from build123d import *

# Parameters (mm, degrees)
SKETCH1_R           = 4
BOSS_EXTRUDE1_DEPTH = 6
BOSS_EXTRUDE2_DEPTH = 6
CIRPATTERN1_COUNT   = 17
SKETCH5_R           = 3
CUT_EXTRUDE1_DEPTH  = 6


with BuildPart() as part:
    # Sketch1 → Boss-Extrude1 (new body)
    with BuildSketch(Plane.XY):
        Circle(SKETCH1_R)
    extrude(amount=BOSS_EXTRUDE1_DEPTH)

    # Sketch3 → Boss-Extrude2 (add)
    with BuildSketch(Plane.XY):
        Polygon((0, 4.768626967), (0.25, 4.768626967), (0.5, 3.968626967), (-0.5, 3.968626967), (-0.25, 4.768626967), align=None)
    boss_extrude2 = extrude(amount=BOSS_EXTRUDE2_DEPTH)

    # CirPattern1: Boss-Extrude2 ×17 about axis
    cirpattern1_axis = Axis((0, 0, 0), (0, 0, 1))
    for i in range(1, CIRPATTERN1_COUNT):
        add(boss_extrude2.rotate(cirpattern1_axis, i * 360 / CIRPATTERN1_COUNT))

    # Sketch5 → Cut-Extrude1 (cut)
    with BuildSketch(Plane.XY):
        Circle(SKETCH5_R)
    extrude(amount=CUT_EXTRUDE1_DEPTH, mode=Mode.SUBTRACT)


solid = part.part
Geometry check sheet. Reference: the model listing, model coordinates, mm. A direction names the side the tool comes from. Give positions to 0.01 mm unless a question says otherwise; leave off trailing zeros. Loops run counter-clockwise (first coordinate to the right, second up) from the corner with the lowest first, then second, coordinate; pieces in that order, holes last.
(1) Release check for a two-part mould opening along Y. For faces 1 (the flat face through (1.928, 3.944, 2.958)), 2 (the flat face through (-1.17, -4.23, 2.96)), 3 (the cylindrical face through (-3, 0, 3)), 4 (the flat face through (0.373, 4.374, 2.958)) record: released by +Y, released by -Y, zero draft, split by the parting line, or undercut.
From the geometry:
face 1: undercut
face 2: released by -Y
face 3: undercut
face 4: released by +Y
(2) Section check A-A on x = 0. Record the cut outline in (y, z), then the cut area to 3 significant figures.
From the geometry:
outline: (-4, 0) - (-3, 0) - (-3, 6) - (-4, 6) - close; (3, 0) - (4.77, 0) - (4.77, 6) - (3, 6) - close
area: 16.6 mm2
(3) Section check B-B on y = -2.5. Record the cut outline in (x, z).
From the geometry:
outline: (-3.83, 0) - (-1.66, 0) - (-1.66, 6) - (-3.83, 6) - close; (1.66, 0) - (3.83, 0) - (3.83, 6) - (1.66, 6) - close
(4) Set-up check for faces 5 (the flat face through (-0.377, 4.363, 2.958)), 6 (the flat face through (4.31, 0.778, 2.958)), 7 (the flat face through (-2.62, -3.52, 2.96)), 8 (the flat face through (-1.927, 3.932, 2.958)): record each of +Z, -Z, +X, -X, +Y, -Y from which the full face is reachable in a straight line by a thin tool's end or side.
From the geometry:
face 5: +Z, -Z, +Y
face 6: +Z, -Z, +X
face 7: +Z, -Z, -X
face 8: +Z, -Z
(5) Depth check by flat-ended pin: pin 1 Ø5.5 at (x, y) = (0, 0) entering from -Z; pin 2 Ø2 at (x, z) = (2, 1.5) entering from +Y; pin 3 Ø1.5 at (y, z) = (-1, 1) entering from +X (3 decimals). Enter the tip coordinate at first touch or a pass-through.
From the geometry:
pin 1: passes through
pin 2: stops at y = 4.54
pin 3: stops at x = 4.655
(6) Section check C-C on y = -3.5. Record the cut outline in (x, z), then the cut area to 3 significant figures.
From the geometry:
outline: (-2.61, 0) - (2.61, 0) - (2.61, 6) - (-2.61, 6) - close
area: 31.4 mm2
(7) Thickness scan on L1, parallel to Y at x = 0, z = 1.8; L2, parallel to Y at x = 4.25, z = 5.65; L3, parallel to X at y = -0.75, z = 1.35 (3 decimals). Record the ranges inside material, lowest first.
From the geometry:
L1: y = -4 to -3, 3 to 4.77
L2: y = -1.55 to -0.8, -0.03 to 0.79, 1.78 to 2.16
L3: x = -4.175 to -2.905, 2.905 to 4.175
